Check sheet for the modelled part. Datum: model origin and axes. Units: mm. Face numbers are marked on the shaded views. A direction names the side the tool comes from. Give positions to 0.01 mm unless a question says otherwise; leave off trailing zeros. Loops run counter-clockwise (first coordinate to the right, second up) from the corner with the lowest first, then second, coordinate; pieces in that order, holes last. Notation, with made-up numbers: (61, 48.5) - (118, 48.5) arc R16 ccw to (118, 64.5) - close; hole circle Ø10 at (-17, 83.5). An arc over 180 degrees is marked (long way). Use CSV: the item, a comma, the result in double quotes.
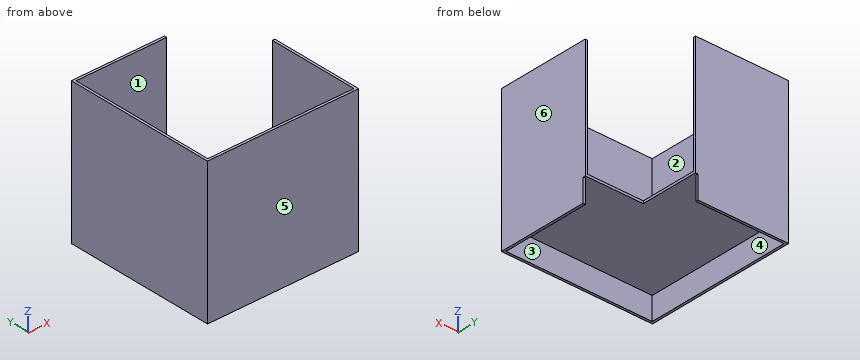
from build123d import *

# Parameters (mm, degrees)
F2_DEPTH  = 15
F3_DEPTH  = 15
F6_DEPTH  = 15
F9_DEPTH  = 15
F11_W     = 910
F11_H     = 875
F12_DEPTH = 15


with BuildPart() as f2:
    # F0 (on Right) → F2 (new body)
    with BuildSketch(Plane.YZ):
        Polygon((-15, -140), (540, -140), (540, 0), (555, 0), (555, 735), (-15, 735), align=None)
    extrude(amount=F2_DEPTH)

    # F1 (on Top) → F3 (join)
    with BuildSketch(Plane.XY):
        Polygon((-895, 0), (0, 0), (0, 555), (-340, 555), (-340, 895), (-895, 895), align=None)
    extrude(amount=F3_DEPTH)

    # F5 (on offset) → F6 (join)
    with BuildSketch(Plane(origin=(-895, 0, 0), x_dir=(0, -1, 0), z_dir=(-1, 0, 0))):
        Polygon((0, -140), (0, 0), (0, 735), (-895, 735), (-895, -140), align=None)
    extrude(amount=F6_DEPTH)

    # F8 (on offset) → F9 (join)
    with BuildSketch(Plane(origin=(0, 895, 0), x_dir=(-1, 0, 0), z_dir=(0, 1, 0))):
        Polygon((355, -140), (910, -140), (910, 735), (340, 735), (340, 0), (355, 0), align=None)
    extrude(amount=F9_DEPTH)

    # F11 (on offset) → F12 (join)
    with BuildSketch(Plane.XZ):
        with Locations((-455, 297.5)):
            Rectangle(F11_W, F11_H)
    extrude(amount=F12_DEPTH)


solid = f2.part
1. Scan lines: line 1 along X through (y, z) = (324.5, 676.5); line 2 along Y through (x, z) = (-695.5, -93.5); line 3 along Z through (x, y) = (-756.5, 799.5). Record each from-to range of solid material in increasing order.
Completed:
line 1,"x = -910 to -895, 0 to 15"
line 2,"y = -15 to 0, 895 to 910"
line 3,"z = 0 to 15"
2. Go/stop test with flat-tipped pins: pin 1 Ø6 at (x, y) = (-277, 280) entering from +Z; pin 2 Ø7.5 at (x, z) = (11, -85) entering from +Y; pin 3 Ø12 at (y, z) = (902, -52.5) entering from +X. Record where each tip stops, or that it passes through.
Completed:
pin 1,"stops at z = 15"
pin 2,"stops at y = 540"
pin 3,"stops at x = -355"
3. Release check for a two-part mould opening along X. For the marked faces 4, 5 and 6 record: released by +X, released by -X, zero draft, split by the parting line, or undercut.
Completed:
face 4,"undercut"
face 5,"zero draft"
face 6,"released by +X"
4. Sectioned sample at B-B, the plane z = 299. Record the boundary of the cut face in (x, y), and give its area (3 significant figures).
Completed:
outline,"(-910, -15) - (15, -15) - (15, 555) - (0, 555) - (0, 0) - (-895, 0) - (-895, 895) - (-340, 895) - (-340, 910) - (-910, 910) - close"
area,"44,200 mm²"
5. Set-up check for the marked faces 1, 2 and 3: record each of +Z, -Z, +X, -X, +Y, -Y from which the full face is reachable in a straight line by a thin tool's end or side.
Completed:
face 1,"+Z, +X"
face 2,"+Z"
face 3,"-Z"
6. Sectioned sample at C-C, the plane y = 380. Record the boundary of the cut face in (x, z).
Completed:
outline,"(-910, -140) - (-895, -140) - (-895, 0) - (0, 0) - (0, -140) - (15, -140) - (15, 735) - (0, 735) - (0, 15) - (-895, 15) - (-895, 735) - (-910, 735) - close"
7. Sectioned sample at A-A, the plane x = -649. Record the boundary of the cut face in (y, z), and give its area (3 significant figures).
Completed:
outline,"(-15, -140) - (0, -140) - (0, 0) - (895, 0) - (895, -140) - (910, -140) - (910, 735) - (895, 735) - (895, 15) - (0, 15) - (0, 735) - (-15, 735) - close"
area,"39,700 mm²"
8. Sectioned sample at D-D, the plane x = -65.5. Record the boundary of the cut face in (y, z).
Completed:
outline,"(-15, -140) - (0, -140) - (0, 0) - (555, 0) - (555, 15) - (0, 15) - (0, 735) - (-15, 735) - close"
